Model file for the job. Use its own axes, mm. Face numbers are marked on the shaded views. Round coordinates to 2 decimals unless told otherwise and drop trailing zeros. Order: outer loops, then holes, each group sorted by start corner. A loop starts at its lowest first (then second) coordinate and runs counter-clockwise, first axis right, second up. Notation, with made-up numbers: (73.5, -23.5) - (117.5, -23.5) arc R17 ccw to (117.5, -15.5) - close; hole circle Ø1 at (36, 43.5). An arc over 180 degrees is marked (long way). Write item = value, one per line.
```python
from build123d import *

# Parameters (mm, degrees)
F0_R     = 27.9199968723
F1_DEPTH = 55.372
F3_R     = 150
F3_R_2   = 75
F4_DEPTH = 100


with BuildPart() as f1:
    # F0 (on Top) → F1 (new body)
    with BuildSketch(Plane.XY):
        with Locations((0, -4.4582164846)):
            Circle(F0_R)
    extrude(amount=F1_DEPTH)


with BuildPart() as f4:
    # F3 (on Top) → F4 (new body)
    with BuildSketch(Plane.XY):
        Circle(F3_R)
        Circle(F3_R_2, mode=Mode.SUBTRACT)
    extrude(amount=F4_DEPTH)


solid = f4.part
```
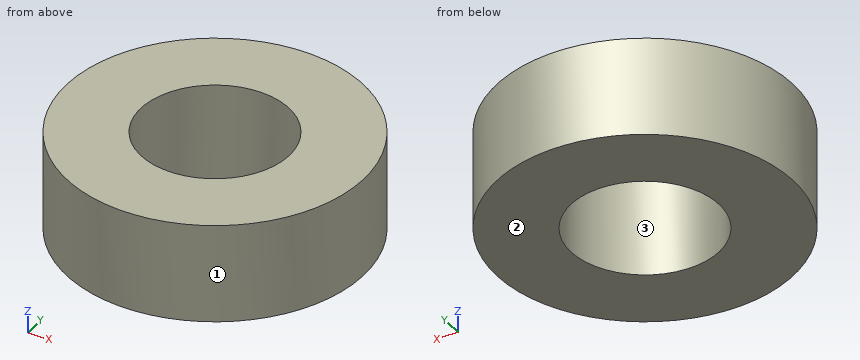
1) Cut at C-C (z = 81). Write the cut outline in (x, y), and give its area (3 significant figures).
Conclusion:
outline = circle Ø300 at (0, 0); hole circle Ø150 at (0, 0)
area = 53,000 mm^2
2) Mould opens along Y. For the marked faces 1, 2 and 3 say: +Y half, -Y half, draft (parallel to the pull), parting line (faces both ways), or undercut.
Conclusion:
face_1 = parting line
face_2 = draft
face_3 = undercut
3) Wall check: line 1 along Y through (x, z) = (0, 78); line 2 along X through (y, z) = (-4, 43.5); line 3 along X through (y, z) = (-64.5, 36). Give the ranges that are in metal, low to high.
Conclusion:
line_1 = -150 to -75, 75 to 150
line_2 = -149.95 to -74.89, 74.89 to 149.95
line_3 = -135.42 to -38.27, 38.27 to 135.42
4) Cut at A-A (x = 0). Write the cut outline in (y, z).
Conclusion:
outline = (-150, 0) - (-75, 0) - (-75, 100) - (-150, 100) - close; (75, 0) - (150, 0) - (150, 100) - (75, 100) - close
5) Flat gauge pins, fed straight in: pin 1 Ø4 at (x, y) = (49, 58.5) entering from -Z; pin 2 Ø4 at (x, z) = (-43.5, 24) entering from -Y; pin 3 Ø10 at (x, z) = (-83.5, 29.5) entering from -Y; pin 4 Ø12 at (y, z) = (37, 77) entering from +X. Where does each tip first touch, or does it go through?
Conclusion:
pin_1 = 0
pin_2 = -144.14
pin_3 = -127.82
pin_4 = 146.76
6) Cut at D-D (y = -115.5). Write the cut outline in (x, z), and give its area (3 significant figures).
Conclusion:
outline = (-95.71, 0) - (95.71, 0) - (95.71, 100) - (-95.71, 100) - close
area = 19,100 mm^2
